```python
from build123d import *
from build123d.topology import SkipClean

# Parameters (mm, degrees)
EXTRUDE_1_DEPTH          = 14
CUT_EXTRUDE_1_DEPTH      = 57.762663785
SKETCH_4_R               = 7
CUT_EXTRUDE_2_DEPTH      = 57.762663785
CUT_EXTRUDE_START        = 6
CUT_EXTRUDE_3_DEPTH      = 51.762663785
SKETCH_7_R               = 20
EXTRUDE_2_DEPTH          = 14
CUT_EXTRUDE_4_DEPTH      = 57.762663785
CUT_EXTRUDE_4_DEPTH_BACK = 57.762663785
SKETCH_6_W               = 36
SKETCH_6_H               = 3
CUT_EXTRUDE_5_DEPTH      = 57.098128311
CUT_EXTRUDE_5_DEPTH_BACK = 57.098128311
SKETCH_9_R               = 12.5
FILLET_1_R               = 10
FILLET_4_R               = 2


with BuildPart() as part:
    # 草图2 → 凸台-拉伸1 (new body)
    with BuildSketch(Plane(origin=(0, 0, 0), x_dir=(1, 0, 0), z_dir=(0, 1, 0))):
        with BuildLine():
            Line((7.857142857, 23.733211037), (39.4, 13.290598181))
            ThreePointArc((39.4, 13.290598181), (49, 0), (39.4, -13.290598181))
            Line((39.4, -13.290598181), (7.857142857, -23.733211037))
            ThreePointArc((7.857142857, -23.733211037), (0, -25), (-7.857142857, -23.733211037))
            Line((-7.857142857, -23.733211037), (-39.4, -13.290598181))
            ThreePointArc((-39.4, -13.290598181), (-49, 0), (-39.4, 13.290598181))
            Line((-39.4, 13.290598181), (-7.857142857, 23.733211037))
            ThreePointArc((-7.857142857, 23.733211037), (0, 25), (7.857142857, 23.733211037))
        make_face()
    extrude(amount=EXTRUDE_1_DEPTH)

    # 草图3 → 切除-拉伸1 (cut, symmetric)
    with BuildSketch(Plane.XY):
        Polygon((-255.331422272, -6.84338141), (-49, 10), (0, 14), (206.331422272, 30.84338141), (172.644659452, 443.506225953), (-289.018185091, 405.819463133), align=None)
    cut_extrude_1 = extrude(amount=CUT_EXTRUDE_1_DEPTH, both=True, mode=Mode.SUBTRACT)

    # 镜向1: 切除-拉伸1 across plane
    add(cut_extrude_1.mirror(Plane(origin=(0, 0, 0), x_dir=(0, 0, 1), z_dir=(1, 0, 0))), mode=Mode.SUBTRACT)

    # 草图4 → 切除-拉伸2 (cut, through all)
    with BuildSketch(Plane.XZ):
        with Locations(Location((-35, 0, 0), (0, 0, 270))):
            Circle(SKETCH_4_R)
        with Locations((35, 0)):
            Circle(SKETCH_4_R)
    extrude(amount=-CUT_EXTRUDE_2_DEPTH, mode=Mode.SUBTRACT)

    # 草图5 → 切除-拉伸3 (cut, through all)
    with BuildSketch(Plane(origin=(0, 0, 0), x_dir=(1, 0, 0), z_dir=(0, 1, 0)).offset(CUT_EXTRUDE_START)):
        with BuildLine():
            Line((-38.142857143, -9.493284415), (-14.26843517, -17.397176719))
            ThreePointArc((-14.26843517, -17.397176719), (-22.5, 0), (-14.26843517, 17.397176719))
            Line((-14.26843517, 17.397176719), (-38.142857143, 9.493284415))
            ThreePointArc((-38.142857143, 9.493284415), (-45, 0), (-38.142857143, -9.493284415))
        make_face()
    cut_extrude_3 = extrude(amount=CUT_EXTRUDE_3_DEPTH, mode=Mode.SUBTRACT)

    # 镜向2: 切除-拉伸3 across plane
    add(cut_extrude_3.mirror(Plane(origin=(0, 0, 0), x_dir=(0, 0, 1), z_dir=(1, 0, 0))), mode=Mode.SUBTRACT)

    # 草图7 → 凸台-拉伸2 (add)
    with BuildSketch(Plane(origin=(0, 0, 0), x_dir=(1, 0, 0), z_dir=(0, 1, 0))):
        Circle(SKETCH_7_R)
    extrude(amount=EXTRUDE_2_DEPTH)

    # 草图6 → 切除-拉伸4 (cut, two sides: drawn at the far end of the back side and taken through both)
    with BuildSketch(Plane.XY.offset(-CUT_EXTRUDE_4_DEPTH_BACK)):
        with Locations((0, 1.5)):
            Rectangle(SKETCH_6_W, SKETCH_6_H)
    extrude(amount=CUT_EXTRUDE_4_DEPTH + CUT_EXTRUDE_4_DEPTH_BACK, mode=Mode.SUBTRACT)

    # 草图8 → 切除-旋转3 (revolve, cut)
    with SkipClean():  # the faces are left unmerged after this step: merging them gives an invalid solid
        with BuildSketch(Plane.XY):
            with BuildLine():
                ThreePointArc((0, 11.94870108), (9.058253519, 12.463180114), (18, 14))
                Line((18, 14), (0, 14))
                Line((0, 14), (0, 11.94870108))
            make_face()
            with BuildLine():
                Line((0, 11.94870108), (0, 14))
                Line((0, 14), (-18, 14))
                ThreePointArc((-18, 14), (-9.058253519, 12.463180114), (0, 11.94870108))
            make_face()
        revolve(axis=Axis((0, -0.298834831, 0), (0, 1, 0)), mode=Mode.SUBTRACT)
    add(part.part.scale(1), mode=Mode.REPLACE)  # the faces are merged on a copy

    # 草图9 → 切除-拉伸5 (cut, two sides: drawn at the far end of the back side and taken through both)
    with BuildSketch(Plane.XZ.offset(-3).offset(-CUT_EXTRUDE_5_DEPTH_BACK)):
        Circle(SKETCH_9_R)
    extrude(amount=CUT_EXTRUDE_5_DEPTH + CUT_EXTRUDE_5_DEPTH_BACK, mode=Mode.SUBTRACT)

    # 圆角1
    # the kernel refuses this fillet: 10 mm, written as the material it takes off along each edge
    with BuildSketch(Plane(origin=(0, 14, 17.959183673), x_dir=(0.9966846158226077, -0.08136200945491137, 0), z_dir=(0, 0, 1))) as fillet_1_piece_1_section:
        with BuildLine():
            CenterArc((FILLET_1_R * 0.0816326530612, -FILLET_1_R), FILLET_1_R, 90, 9.333716743)
            Line((-FILLET_1_R * 0.080551873211, -FILLET_1_R * 0.0132395531651), (0, 0))
            Line((0, 0), (FILLET_1_R * 0.0816326530612, 0))
        make_face()
    fillet_1_piece_1 = extrude(amount=9.081632653, mode=Mode.PRIVATE)
    fillet_1_piece_1 = fillet_1_piece_1 - Plane(origin=(0, 13.973401813, 0), x_dir=(1, 0, 0), z_dir=(0, -1, 0)) * Cylinder(20, 22, mode=Mode.PRIVATE)
    add(fillet_1_piece_1, mode=Mode.SUBTRACT)
    with BuildSketch(Plane(origin=(0, 14, -27.040816327), x_dir=(0.9966846158226077, -0.08136200945491137, 0), z_dir=(0, 0, 1))) as fillet_1_piece_2_section:
        with BuildLine():
            CenterArc((FILLET_1_R * 0.0816326530612, -FILLET_1_R), FILLET_1_R, 90, 9.333716743)
            Line((-FILLET_1_R * 0.080551873211, -FILLET_1_R * 0.0132395531651), (0, 0))
            Line((0, 0), (FILLET_1_R * 0.0816326530612, 0))
        make_face()
    fillet_1_piece_2 = extrude(amount=9.081632653, mode=Mode.PRIVATE)
    fillet_1_piece_2 = fillet_1_piece_2 - Plane(origin=(0, 13.973401813, 0), x_dir=(1, 0, 0), z_dir=(0, -1, 0)) * Cylinder(20, 22, mode=Mode.PRIVATE)
    add(fillet_1_piece_2, mode=Mode.SUBTRACT)

    # 圆角4
    fillet_4_edges = [part.edges().sort_by_distance(p)[0] for p in [
        (26.205646157, 6, 13.445230567),
        (45, 6, 0),
        (-26.205646157, 6, 13.445230567),
        (-45, 6, 0),
        (-14.26843517, 9.417614891, 17.397176719),
        (14.26843517, 9.417614891, 17.397176719),
        (26.205646157, 6, -13.445230567),
        (14.26843517, 9.417614891, -17.397176719),
        (22.5, 6, 0),
        (-14.26843517, 9.417614891, -17.397176719),
        (-22.5, 6, 0),
        (-26.205646157, 6, -13.445230567),
    ]]
    fillet(fillet_4_edges, radius=FILLET_4_R)


solid = part.part
```
CAD build for the part. Positions are in the model's coordinates, mm. A direction names the side the tool comes from. Coordinates: 2 decimals unless noted, no trailing zeros. Order: outer loops, then holes, each group sorted by start corner. A loop starts at its lowest first (then second) coordinate and runs counter-clockwise, first axis right, second up. Notation, with made-up numbers: (83.25, 76.25) -> (104.25, 76.25) arc R14 cw to (104.25, 102.25) -> close; hole circle Ø1 at (6.5, 80.25). An arc over 180 degrees is marked (long way). Use one line per item in the form item = value. Start each with the question number.
1) Pull direction Z, two halves, no side cores. Call faces 1 (the cylindrical face through (45, 9, 0)), 2 (the cylindrical face through (0, 8, -25)), 3 (the flat face through (23.85, 6.59, 18.44)), 4 (the flat face through (21.45, 12.25, 1.97)): +Z half, -Z half, draft (parallel to the pull), parting line (faces both ways), or undercut.
2) Band-saw the part on C-C on z = -3.5. State how many separate pieces and enclosed holes the cut face has, then the cut area to 3 significant figures.
3) Drop flat-ended pins along their axis: pin 1 (6.5 mm diameter, centred on x = -32, z = 0.5, fed in from +Y); pin 2 (6 mm diameter, centred on x = 24.5, y = 8.5, fed in from +Z); pin 3 (0.9 mm diameter, centred on y = 1.5, z = 9, fed in from +X); pin 4 (3.5 mm diameter, centred on y = 2, z = 7.5, fed in from -X). Give the stop position or say it passes through.
4) Band-saw the part on B-B on x = -10.5. Give the cut face in (y, z), then the cut area to 3 significant figures.
5) Drill centre lines: L1, parallel to X at y = 9.25, z = 0; L2, parallel to Y at x = -24, z = -12; L3, parallel to Z at x = -29, y = 9. Where is each one in solid material? Low to high. Write a range as [from, to].
6) Band-saw the part on A-A on y = 5. Give the cut face in (x, z), then the cut area to 3 significant figures.
7) Tool access for faces 5 (the cylindrical face through (29.41, 6.57, 11.75)), 6 (the flat face through (-12, 3, 5)), 7 (the flat face through (-21.45, 12.25, 1.97)): list every direction of +Z, -Z, +X, -X, +Y, -Y with a clear straight run to the whole face (end or side of a thin tool).
Entries:
q1.face_1 = undercut
q1.face_2 = -Z half
q1.face_3 = +Z half
q1.face_4 = draft
q2.separate_pieces = 4
q2.enclosed_holes = 0
q2.area = 444 mm2
q3.pin_1 = through
q3.pin_2 = 19.22
q3.pin_3 = 46.09
q3.pin_4 = -47.76
q4.outline = (3, -22.86) -> (13.14, -22.86) -> (13.14, -17.02) -> (14, -17.02) -> (14, -14.62) arc R79.31 cw to (12.93, -6.78) -> (3, -6.78) -> close; (3, 6.78) -> (12.93, 6.78) arc R79.31 cw to (14, 14.62) -> (14, 17.02) -> (13.14, 17.02) -> (13.14, 22.86) -> (3, 22.86) -> close
q4.area = 334 mm2
q5.L1 = [-49, -45], [-22.5, -12.5], [12.5, 22.5], [45, 49]
q5.L2 = [0, 6]
q5.L3 = [-16.73, -12.52], [12.52, 16.73]
q6.outline = (-39.4, -13.29) -> (-7.86, -23.73) arc R25 ccw to (7.86, -23.73) -> (39.4, -13.29) arc R14 ccw to (39.4, 13.29) -> (7.86, 23.73) arc R25 ccw to (-7.86, 23.73) -> (-39.4, 13.29) arc R14 ccw to start; hole circle Ø14 at (-35, 0); hole circle Ø25 at (0, 0); hole circle Ø14 at (35, 0)
q6.area = 2,680 mm2
q7.face_5 = +Y
q7.face_6 = +Z, -Z, -Y
q7.face_7 = -X, +Y
